from build123d import *

# Parameters (mm, degrees)
SKETCH1_W                = 73
SKETCH1_H                = 59.5
GREEN_PCB_DEPTH          = 1.6
SKETCH2_W                = 57.5
SKETCH2_H                = 41
BLUE_PCB_DEPTH           = 2.1
SKETCH3_W                = 45
SKETCH3_H                = 16
SKETCH3_W_2              = 15
SKETCH3_H_2              = 8
CLAMP_AREA_DEPTH         = 0.001
SKETCH4_W                = 7.5
SKETCH4_H                = 7.8
USB_PORT_DEPTH           = 2.6
USB_BODY_DEPTH           = 3.5
SKETCH7_R                = 3.5
USB_TENSION_RELIEF_DEPTH = 6
SKETCH8_R                = 2
USB_CORD_DEPTH           = 15
SKETCH9_R                = 5.5
MONA_LISA_ANTENNA_DEPTH  = 0.001
LPATTERN1_COUNT          = 2
LPATTERN1_PITCH          = 20.5
LPATTERN2_COUNT          = 2
LPATTERN2_PITCH          = 12.5


with BuildPart() as part:
    # Sketch1 → Green PCB (new body)
    with BuildSketch(Plane.XY):
        with Locations((-36.5, 29.75)):
            Rectangle(SKETCH1_W, SKETCH1_H)
    extrude(amount=GREEN_PCB_DEPTH)

    # Sketch2 → Blue PCB (add)
    with BuildSketch(Plane.XY.offset(1.6)):
        with Locations((-74.25, 25)):
            Rectangle(SKETCH2_W, SKETCH2_H)
    extrude(amount=BLUE_PCB_DEPTH)

    # Sketch3 → Clamp Area (add)
    with BuildSketch(Plane.XY.offset(1.6)):
        with Locations((-22.5, 51.5)):
            Rectangle(SKETCH3_W, SKETCH3_H)
        with Locations((-37.5, 4)):
            Rectangle(SKETCH3_W_2, SKETCH3_H_2)
    extrude(amount=CLAMP_AREA_DEPTH)

    # Sketch4 → USB Port (add)
    with BuildSketch(Plane.XY.offset(1.6)):
        with Locations((-6.25, 0.6)):
            Rectangle(SKETCH4_W, SKETCH4_H)
    usb_port = extrude(amount=USB_PORT_DEPTH)

    # Sketch5 → USB Body (add, symmetric)
    with BuildSketch(Plane.XY.offset(2.9)):
        with BuildLine():
            Line((-11.75, -3.3), (-0.75, -3.3))
            Line((-0.75, -3.3), (-0.75, -18.8))
            ThreePointArc((-0.75, -18.8), (-6.25, -24.3), (-11.75, -18.8))
            Line((-11.75, -18.8), (-11.75, -3.3))
        make_face()
    usb_body = extrude(amount=USB_BODY_DEPTH, both=True)

    # Sketch7 → USB Tension Relief (add, symmetric)
    with BuildSketch(Plane(origin=(0, -24.3, 0), x_dir=(-1, 0, 0), z_dir=(0, -1, 0))):
        with Locations(Location((6.25, -2.9, 0), (0, 0, 90))):
            Circle(SKETCH7_R)
    usb_tension_relief = extrude(amount=USB_TENSION_RELIEF_DEPTH, both=True)

    # Sketch8 → USB Cord (add)
    with BuildSketch(Plane.XZ.offset(30.3)):
        with Locations(Location((-6.25, 2.9, 0), (0, 0, 270))):
            Circle(SKETCH8_R)
    usb_cord = extrude(amount=USB_CORD_DEPTH)

    # Sketch9 → Mona Lisa Antenna (add)
    with BuildSketch(Plane(origin=(0, 0, 1.6), x_dir=(-1, 0, 0), z_dir=(0, 0, -1))):
        with Locations(Location((88.2, 35.25, 0), (0, 0, 180))):
            Circle(SKETCH9_R)
        Polygon((85.066571319, 38.121258382), (89.389314163, 36.547908657), (91.333428681, 32.378741618), (87.010685837, 33.952091343), align=None, mode=Mode.SUBTRACT)
    mona_lisa_antenna = extrude(amount=MONA_LISA_ANTENNA_DEPTH)

    # LPattern1: Mona Lisa Antenna ×2
    with Locations(*[(0, -i * LPATTERN1_PITCH, 0) for i in range(1, LPATTERN1_COUNT)]):
        add(mona_lisa_antenna)

    # LPattern2: USB Port, USB Body, USB Tension Relief, USB Cord ×2
    with Locations(*[(-i * LPATTERN2_PITCH, 0, 0) for i in range(1, LPATTERN2_COUNT)]):
        add(usb_port)
        add(usb_body)
        add(usb_tension_relief)
        add(usb_cord)


solid = part.part
Design review of the part built by this model. Coordinates are the model's own, in mm. A direction names the side the tool comes from. Give positions to 0.01 mm unless a question says otherwise; leave off trailing zeros. Order: outer loops, then holes, each group sorted by start corner. A loop starts at its lowest first (then second) coordinate and runs counter-clockwise, first axis right, second up. Notation, with made-up numbers: (78.5, -38.75) - (89.5, -38.75) arc R22 ccw to (89.5, -15.75) - close; hole circle Ø3 at (7.25, 14). An arc over 180 degrees is marked (long way). Write item = value, one per line. Start each with the question number.
Q1. Clearance check with flat-ended pins moving along their axes: pin 1 Ø4 at (x, y) = (-70, 37.5) entering from +Z; pin 2 Ø8 at (x, y) = (-20.5, 49) entering from +Z; pin 3 Ø0.5 at (x, z) = (-33, 1) entering from -Y. State where each tip first meets the part, or that it passes through.
Q2. To check wall thickness, follow L1, parallel to X at y = -3.5, z = 3.75; L2, parallel to X at y = -38.5, z = 3; L3, parallel to Y at x = -83.5, z = 2.25. State the ranges of each line that lie inside material, in increasing order. Write a range as from..to.
Q3. Tool access review of faces 1 (the face through (-6, 1, 4.2)), 2 (the face through (-15, 1, 3)), 3 (the face through (-88, 38, 1.599)): name each direction out of +Z, -Z, +X, -X, +Y, -Y from which nothing blocks a thin tool from reaching the whole face with its end or side.
Q4. Mouldability with a two-part tool opening along X and no side actions: class faces 4 (the face through (-23.7, -21.2, 2.9)), 5 (the face through (-11.2, -21.2, 2.9)), 6 (the face through (-88, 25, 1.6)) as released by +X, released by -X, zero draft, split by the parting line, or undercut.
Q5. We need section A-A on y = -10.5. State the section outline as (x, z) points.
Q6. We need section D-D on y = -38. State the section outline as (x, z) points.
Working result:
q1.pin_1 = 3.7
q1.pin_2 = 1.6
q1.pin_3 = 0
q2.L1 = -24.25..-13.25, -11.75..-0.75
q2.L2 = -20.75..-16.75, -8.25..-4.25
q2.L3 = 4.5..45.5
q3.face_1 = +Z, +X, -X, +Y
q3.face_2 = +Z, +Y
q3.face_3 = -Z, -X, +Y, -Y
q4.face_4 = released by -X
q4.face_5 = undercut
q4.face_6 = zero draft
q5.outline = (-24.25, -0.6) - (-13.25, -0.6) - (-13.25, 6.4) - (-24.25, 6.4) - close; (-11.75, -0.6) - (-0.75, -0.6) - (-0.75, 6.4) - (-11.75, 6.4) - close
q6.outline = circle Ø4 at (-18.75, 2.9); circle Ø4 at (-6.25, 2.9)
